Read the model definition and answer for the solid it produces. Units are mm, in the model's axes. A direction names the side the tool comes from. Give positions to 0.01 mm unless a question says otherwise; leave off trailing zeros. Order: outer loops, then holes, each group sorted by start corner. A loop starts at its lowest first (then second) coordinate and runs counter-clockwise, first axis right, second up. Notation, with made-up numbers: (-31.75, 62.25) - (19.25, 62.25) arc R30 ccw to (19.25, 86.25) - close; hole circle Ø4 at (83.5, 32). An arc over 180 degrees is marked (long way). Answer as CSV lines item,"result". Start each with the question number.
from build123d import *

# Parameters (mm, degrees)
SKETCH1_R                            = 19.05
SKETCH1_R_2                          = 12.7
BOSS_EXTRUDE1_DEPTH                  = 76.2
SKETCH2_W                            = 10.668
SKETCH2_H                            = 12.7
BOSS_EXTRUDE2_DEPTH                  = 12.7
BOSS_EXTRUDE2_DIRECTION_2_REACH      = 89.298
BOSS_EXTRUDE2_DIRECTION_2_END_RADIUS = 19.05
SKETCH3_R                            = 19.05
BOSS_EXTRUDE3_DEPTH                  = 2.032
SKETCH4_W                            = 5.08
SKETCH4_H                            = 35.306
CUT_EXTRUDE1_DEPTH                   = 87.551781172
BOSS_EXTRUDE4_REACH                  = 105.578
BOSS_EXTRUDE4_END_RADIUS             = 19.05
SKETCH7_W                            = 35.56
SKETCH7_H                            = 10.16
F_8_0_199_DIAMETER_HOLE1_D           = 5.0546


with BuildPart() as part:
    # Sketch1 → Boss-Extrude1 (new body)
    with BuildSketch(Plane(origin=(0, 0, 0), x_dir=(1, 0, 0), z_dir=(0, 1, 0))):
        with Locations(Location((0, 0, 0), (0, 0, 270))):
            Circle(SKETCH1_R)
        with Locations(Location((0, 0, 0), (0, 0, 270))):
            Circle(SKETCH1_R_2, mode=Mode.SUBTRACT)
    extrude(amount=-BOSS_EXTRUDE1_DEPTH)

    # Sketch2 → Boss-Extrude2 (add)
    with BuildSketch(Plane.XY.offset(19.05)):
        with Locations((5.334, -6.35)):
            Rectangle(SKETCH2_W, SKETCH2_H)
        with Locations((5.334, -41.656)):
            Rectangle(SKETCH2_W, SKETCH2_H)
    extrude(amount=BOSS_EXTRUDE2_DEPTH)

    # Boss-Extrude2 direction 2: up to this cylinder (the profile starts outside it)
    boss_extrude2_direction_2_end = Plane(origin=(0, -24.003, 0), z_dir=(0, 1, 0)) * Cylinder(BOSS_EXTRUDE2_DIRECTION_2_END_RADIUS, 253.002, mode=Mode.PRIVATE)
    # Sketch2 → Boss-Extrude2 direction 2 (add, up to the surface)
    with BuildSketch(Plane.XY.offset(19.05), mode=Mode.PRIVATE) as boss_extrude2_direction_2_sk1:
        with Locations((5.334, -6.35)):
            Rectangle(SKETCH2_W, SKETCH2_H)
    boss_extrude2_direction_2_tool1 = extrude(boss_extrude2_direction_2_sk1.sketch, amount=-BOSS_EXTRUDE2_DIRECTION_2_REACH, mode=Mode.PRIVATE) - boss_extrude2_direction_2_end
    add(boss_extrude2_direction_2_tool1.solids().sort_by_distance((5.334, -6.35, 19.05))[0])
    # Sketch2 → Boss-Extrude2 direction 2 (add, up to the surface)
    with BuildSketch(Plane.XY.offset(19.05), mode=Mode.PRIVATE) as boss_extrude2_direction_2_sk2:
        with Locations((5.334, -41.656)):
            Rectangle(SKETCH2_W, SKETCH2_H)
    boss_extrude2_direction_2_tool2 = extrude(boss_extrude2_direction_2_sk2.sketch, amount=-BOSS_EXTRUDE2_DIRECTION_2_REACH, mode=Mode.PRIVATE) - boss_extrude2_direction_2_end
    add(boss_extrude2_direction_2_tool2.solids().sort_by_distance((5.334, -41.656, 19.05))[0])

    # Sketch3 → Boss-Extrude3 (add)
    with BuildSketch(Plane.XZ.offset(76.2)):
        with Locations(Location((0, 0, 0), (0, 0, 90))):
            Circle(SKETCH3_R)
    extrude(amount=BOSS_EXTRUDE3_DEPTH)

    # Sketch4 → Cut-Extrude1 (cut, through all)
    with BuildSketch(Plane.XY):
        with Locations((-2.54, -24.003)):
            Rectangle(SKETCH4_W, SKETCH4_H)
    extrude(amount=CUT_EXTRUDE1_DEPTH, mode=Mode.SUBTRACT)

    # Sketch6 → Revolve2 (revolve)
    with BuildSketch(Plane.XY, mode=Mode.PRIVATE) as revolve2_sk:
        Polygon((-14.478, -78.232), (-16.51, -90.932), (-19.05, -90.932), (-19.05, -78.232), align=None)
    revolve(revolve2_sk.sketch.rotate(Axis((0, -78.232, 0), (0, -1, 0)), 270), axis=Axis((0, -78.232, 0), (0, -1, 0)))

    # Boss-Extrude4: up to this cylinder (the profile starts outside it)
    boss_extrude4_end = Plane(origin=(0, -10.16, 0), z_dir=(0, 1, 0)) * Cylinder(BOSS_EXTRUDE4_END_RADIUS, 250.256, mode=Mode.PRIVATE)
    # Sketch7 → Boss-Extrude4 (add, up to the surface)
    with BuildSketch(Plane.ZY.offset(19.05), mode=Mode.PRIVATE) as boss_extrude4_sk1:
        with Locations((0, -10.16)):
            Rectangle(SKETCH7_W, SKETCH7_H)
    boss_extrude4_tool1 = extrude(boss_extrude4_sk1.sketch, amount=-BOSS_EXTRUDE4_REACH, mode=Mode.PRIVATE) - boss_extrude4_end
    boss_extrude4 = boss_extrude4_tool1.solids().sort_by_distance((-19.05, -10.16, 0))[0] + boss_extrude4_tool1.solids().sort_by_distance((-19.05, -10.16, 0))[1]
    add(boss_extrude4)

    # Mirror1: Boss-Extrude4 across plane
    add(boss_extrude4.mirror(Plane(origin=(0, 0, 0), x_dir=(0, 0, 1), z_dir=(1, 0, 0))))

    # #8 (0.199) Diameter Hole1 (through all)
    with Locations(Plane.ZY.offset(19.05)):
        with Locations((0, -10.312752813), (12.7, -10.312752813), (-12.7, -10.312752813)):
            Hole(F_8_0_199_DIAMETER_HOLE1_D / 2)


solid = part.part
(1) Section C-C, the plane x = -11.5 is taken. State how many separate pieces and enclosed holes the cut face has, and give its area (3 significant figures).
(2) Section A-A, the plane y = -45 is taken. Write down the section's boundary in (x, z).
(3) Which of the six approach directions +Z, -Z, +X, -X, +Y, -Y give full straight-line access (tool end or side, diameter ignored) to faces 1 (the flat face through (-16, -15.24, 13)), 2 (the flat face through (-13, -10, -17.78)), 3 (the flat face through (-13, -10, 17.78)), 4 (the flat face through (0, -76.2, 0)), 5 (the flat face through (16, -5.08, -14))?
(4) Flat-ended cylindrical pins translate along their axes: pin 1 Ø15 at (y, z) = (-35, 20) entering from -X; pin 2 Ø6.5 at (y, z) = (-10.31, -12.7) entering from -X; pin 3 Ø4.5 at (y, z) = (-10.31, 0) entering from +X (3 decimals); pin 4 Ø7.5 at (y, z) = (-26, 14) entering from +X. Find the tip coordinate at first contact, or state that the pin passes through.
(5) Section D-D, the plane y = -72 is taken. Write down the section's boundary in (x, z).
(6) Straight lines are drawn through the part: line 1 (Y direction, x = 2.5, z = -12.7); line 2 (X direction, y = -14.5, z = 17); line 3 (X direction, y = -50, z = 0). For each, find the intervals that lie inside material, in ascending order. Write a range as [from, to].
(7) Section B-B, the plane y = -20 is taken. Write down the section's boundary in (x, z), and give its area (3 significant figures).
(8) Determine the mould class of faces 6 (the flat face through (0, -78.232, 0)), 7 (the flat face through (5, -35.306, 26)), 8 (the flat face through (13, -10, -17.78)) for opening direction Y: released by +Y, released by -Y, zero draft, split by the parting line, or undercut.
Checks:
1,separate pieces,"1"
1,enclosed holes,"2"
1,area,"1,690 mm²"
2,outline,"(0, 19.05) arc R19.05 ccw (long way) to (10.67, 15.78) - (10.67, 31.75) - (0, 31.75) - close; hole circle Ø25.4 at (0, 0)"
3,face 1,"+Z, -X, -Y"
3,face 2,"-Z, -X, +Y, -Y"
3,face 3,"+Z, -X, +Y, -Y"
3,face 4,"+Y"
3,face 5,"-Z, +X, +Y"
4,pin 1,"stops at x = -14.38"
4,pin 2,"stops at x = -19.05"
4,pin 3,"passes through"
4,pin 4,"stops at x = 16.06"
5,outline,"circle Ø38.1 at (0, 0); hole circle Ø25.4 at (0, 0)"
6,line 1,"y = [-78.23, -12.84], [-7.79, 0]"
6,line 2,"x = [-19.05, -5.08], [0, 19.05]"
6,line 3,"x = [-19.05, -12.7], [12.7, 19.05]"
7,outline,"(-5.08, 11.64) - (-5.08, 18.36) arc R19.05 ccw (long way) to (0, 19.05) - (0, 12.7) arc R12.7 cw (long way) to start"
7,area,"601 mm²"
8,face 6,"released by -Y"
8,face 7,"undercut"
8,face 8,"zero draft"
